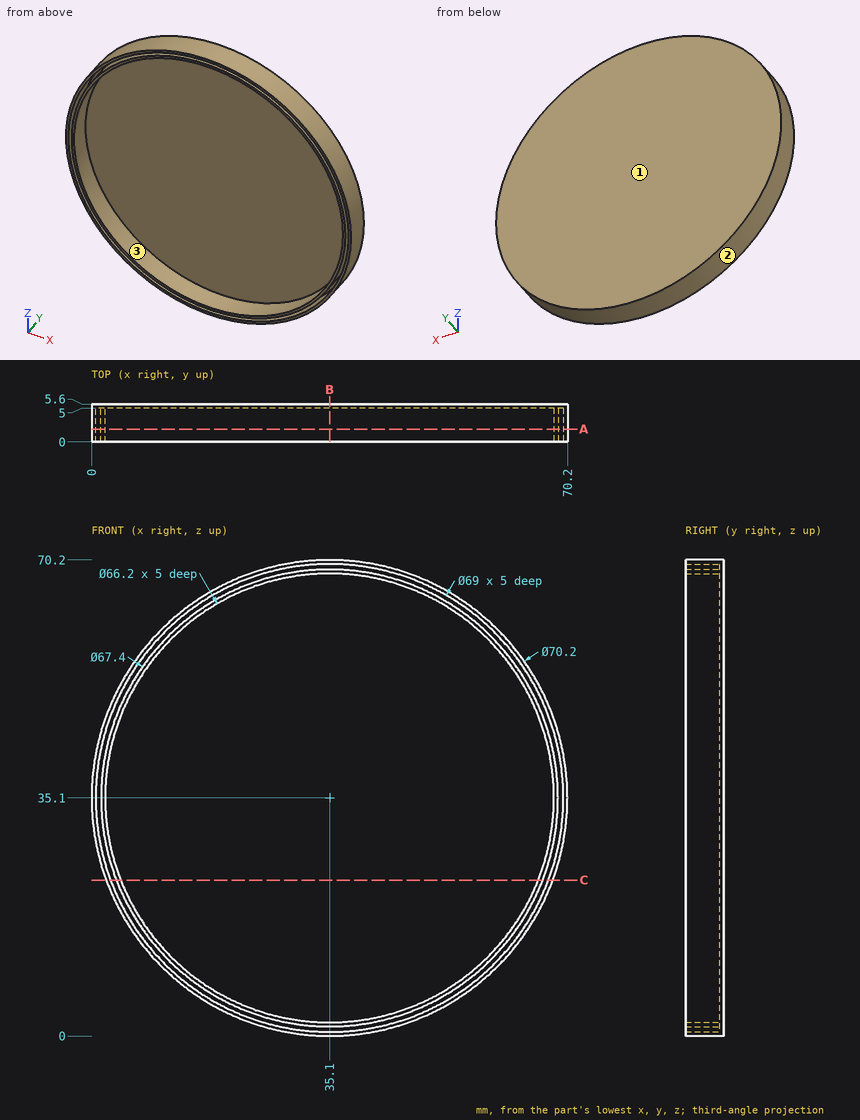
Verification items for this drawing (mm, ordinates from the low corner). Coordinates: 2 decimals unless noted, no trailing zeros. Order: outer loops, then holes, each group sorted by start corner. A loop starts at its lowest first (then second) coordinate and runs counter-clockwise, first axis right, second up. Notation, with made-up numbers: M -17.75,38 L 8.25,38 A5 ccw 8.25,45 Z; hole C 71,12 d7. An arc over 180 degrees is marked long. Use CSV: the item, a comma, the result in double quotes.
Item 1: Mould release check, pull along Z, two halves, no side actions. Record for the marked faces 1, 2 and 3: pulls with the +Z half, pulls with the -Z half, needs draft (parallel to the pull), parting line crosses it, or undercut.
Returned:
face 1,"needs draft"
face 2,"parting line crosses it"
face 3,"undercut"
Item 2: Cross-section at B-B on x = 35.1. Record the cut outline in (y, z).
Returned:
outline,"M 0,0 L 5.6,0 L 5.6,70.2 L 0,70.2 L 0,69.6 L 5,69.6 L 5,68.8 L 0,68.8 L 0,68.2 L 5,68.2 L 5,2 L 0,2 L 0,1.4 L 5,1.4 L 5,0.6 L 0,0.6 Z"
Item 3: Cross-section at C-C on z = 23. Record the cut outline in (x, y), then the cut area to 3 significant figures.
Returned:
outline,"M 2.15,0 L 2.79,0 L 2.79,5 L 3.65,5 L 3.65,0 L 4.29,0 L 4.29,5 L 65.91,5 L 65.91,0 L 66.55,0 L 66.55,5 L 67.41,5 L 67.41,0 L 68.05,0 L 68.05,5.6 L 2.15,5.6 Z"
area,"52.4 mm2"
Item 4: Cross-section at A-A on y = 1.9. Record the cut outline in (x, z), then the cut area to 3 significant figures.
Returned:
outline,"C 35.1,35.1 d70.2; C 35.1,35.1 d67.4; hole C 35.1,35.1 d69; hole C 35.1,35.1 d66.2"
area,"257 mm2"
Item 5: Thickness scan on line 1 along Z through (x, y) = (35.1, 3.7); line 2 along Z through (x, y) = (49.5, 1.85); line 3 along X through (y, z) = (1.4, 61). Record the ranges inside material, lowest first.
Returned:
line 1,"z = 0 to 0.6, 1.4 to 2, 68.2 to 68.8, 69.6 to 70.2"
line 2,"z = 3.09 to 3.75, 4.63 to 5.3, 64.9 to 65.57, 66.45 to 67.11"
line 3,"x = 11.41 to 12.31, 13.54 to 14.49, 55.71 to 56.66, 57.89 to 58.79"
Item 6: Gauge pin test, flat ends, axial feed: pin 1 Ø3 at (x, y) = (40, 3.5) entering from -Z; pin 2 Ø1 at (x, y) = (28, 1.5) entering from -Z; pin 3 Ø1.5 at (x, z) = (39, 20) entering from -Y. Record the tip position at first contact, or that the pin passes through.
Returned:
pin 1,"stops at z = 0.17"
pin 2,"stops at z = 0.63"
pin 3,"stops at y = 5"
